```python
from build123d import *

# Parameters (mm, degrees)
MAIN_DEPTH              = 10
ESQUISSE5_R             = 3
ENL_V_MAT_EXTRU_1_DEPTH = 1
ESQUISSE6_R             = 1.6
ENL_V_MAT_EXTRU_2_DEPTH = 5


with BuildPart() as part:
    # Esquisse1 → Main (new body)
    with BuildSketch(Plane.XY):
        Polygon((0, 5), (3.55, 5), (3.55, 6), (6.45, 6), (6.45, 5), (10, 5), (10, 8.55), (9, 8.55), (9, 11.45), (10, 11.45), (10, 15), (13, 15), (13, 0), (0, 0), align=None)
    extrude(amount=MAIN_DEPTH)

    # Esquisse4 → Fraisage pour vis à tête fraisée (100) #01 (revolve, cut)
    with BuildSketch(Plane(origin=(5, 5, 5), x_dir=(0, 0, 1), z_dir=(1, 0, 0))):
        Polygon((0, 0), (0, 5), (1.6, 5), (1.6, 1.174739484), (3, 0), align=None)
    revolve(axis=Axis((5, 11.35, 5), (0, -1, 0)), mode=Mode.SUBTRACT)

    # Esquisse5 → Enlèv. mat.-Extru.1 (cut)
    with BuildSketch(Plane(origin=(0, 6, 0), x_dir=(1, 0, 0), z_dir=(0, 1, 0))):
        with Locations((5, -5)):
            Circle(ESQUISSE5_R)
    extrude(amount=-ENL_V_MAT_EXTRU_1_DEPTH, mode=Mode.SUBTRACT)

    # Esquisse6 → Enlèv. mat.-Extru.2 (cut, through all)
    with BuildSketch(Plane.ZY.offset(-9)):
        with Locations((5, 10)):
            Circle(ESQUISSE6_R)
    extrude(amount=-ENL_V_MAT_EXTRU_2_DEPTH, mode=Mode.SUBTRACT)


solid = part.part
```
Work out the finished part from the listing and answer in its coordinate system (mm). A direction names the side the tool comes from. Give positions to 0.01 mm unless a question says otherwise; leave off trailing zeros. Order: outer loops, then holes, each group sorted by start corner. A loop starts at its lowest first (then second) coordinate and runs counter-clockwise, first axis right, second up.
1. Each of these flat-tipped pins is pushed along its axis until it touches: P1, Ø1.8, axis at y = 14, z = 6, coming from the -X side; P2, Ø1, axis at x = 2, z = 5.5, coming from the -Y side; P3, Ø2, axis at y = 6.5, z = 3, coming from the -X side; P4, Ø2.5, axis at x = 5.5, z = 9.5, coming from the +Y side. Where does it stop, or does it pass through?
Result sheet:
P1: stops at x = 10
P2: stops at y = 0
P3: stops at x = 3.55
P4: stops at y = 6
2. Section D-D, the plane x = 5 is taken. Determine the outline of the cut face in (y, z).
Result sheet:
outline: (0, 0) - (6, 0) - (6, 2) - (5, 2) - (3.83, 3.4) - (0, 3.4) - close; (0, 6.6) - (3.83, 6.6) - (5, 8) - (6, 8) - (6, 10) - (0, 10) - close
3. Section B-B, the plane z = 5 is taken. Determine the outline of the cut face in (x, y), and give its area (3 significant figures).
Result sheet:
outline: (0, 0) - (3.4, 0) - (3.4, 3.83) - (2, 5) - (0, 5) - close; (6.6, 0) - (13, 0) - (13, 8.4) - (10, 8.4) - (10, 5) - (8, 5) - (6.6, 3.83) - close; (10, 11.6) - (13, 11.6) - (13, 15) - (10, 15) - close
area: 67.8 mm2
4. Straight lines are drawn through the part: L1, parallel to X at y = 1, z = 5; L2, parallel to Z at x = 5, y = 0.85; L3, parallel to Y at x = 11.2, z = 5. For each, find the intervals that lie inside material, in ascending order.
Result sheet:
L1: x = 0 to 3.4, 6.6 to 13
L2: z = 0 to 3.4, 6.6 to 10
L3: y = 0 to 8.4, 11.6 to 15
5. For faces 4 (the flat face through (9, 5, 5)), 5 (the flat face through (5, 6, 1)), 6 (the flat face through (6.45, 5.5, 8.8)), determine the directions among +Z, -Z, +X, -X, +Y, -Y from which every point of the face is accessible in a straight line to the end or side of a thin tool.
Result sheet:
face 4: +Z, -Z
face 5: +Z, -Z, -X, +Y
face 6: +Z, -Z, +Y
6. The mould has two halves that part along Z. Classify faces 1 (the cylindrical face through (3.414, 1.939, 4.792)), 2 (the cylindrical face through (5, 5.5, 2)), 3 (the flat face through (9.5, 8.55, 7.8)): released by +Z, released by -Z, zero draft, split by the parting line, or undercut.
Result sheet:
face 1: undercut
face 2: undercut
face 3: zero draft
7. Section A-A, the plane y = 10 is taken. Determine the outline of the cut face in (x, z), and give its area (3 significant figures).
Result sheet:
outline: (9, 0) - (13, 0) - (13, 3.4) - (9, 3.4) - close; (9, 6.6) - (13, 6.6) - (13, 10) - (9, 10) - close
area: 27.2 mm2
8. Section C-C, the plane x = 11.75 is taken. Determine the outline of the cut face in (y, z).
Result sheet:
outline: (0, 0) - (15, 0) - (15, 10) - (0, 10) - close; hole circle Ø3.2 at (10, 5)
